from build123d import *

# Parameters (mm, degrees)
SKETCH2_W           = 200
SKETCH2_H           = 200
SKETCH2_R           = 60
BOSS_EXTRUDE1_DEPTH = 12
BOSS_EXTRUDE2_START = -2
SKETCH3_R           = 40
SKETCH3_R_2         = 26
BOSS_EXTRUDE2_DEPTH = 2


with BuildPart() as part:
    # Sketch1 → Revolve1 (revolve)
    with BuildSketch(Plane(origin=(0, 0, 0), x_dir=(-1, 0, 0), z_dir=(0, 0, -1)), mode=Mode.PRIVATE) as revolve1_sk:
        with BuildLine():
            Line((-40, 4), (-40, -8))
            Line((-40, -8), (-49.4043, -8))
            ThreePointArc((-49.4043, -8), (-52.5, -6.965718833), (-55.5957, -8))
            Line((-55.5957, -8), (-60, -8))
            Line((-60, -8), (-60, 4))
            Line((-60, 4), (-55.5957, 4))
            ThreePointArc((-55.5957, 4), (-52.5, 2.965718833), (-49.4043, 4))
            Line((-49.4043, 4), (-40, 4))
        make_face()
    revolve(revolve1_sk.sketch.rotate(Axis((0, 0, 0), (0, 1, 0)), 270), axis=Axis((0, 0, 0), (0, 1, 0)))

    # Sketch2 → Boss-Extrude1 (add)
    with BuildSketch(Plane(origin=(0, 4, 0), x_dir=(1, 0, 0), z_dir=(0, 1, 0))):
        Rectangle(SKETCH2_W, SKETCH2_H)
        Circle(SKETCH2_R, mode=Mode.SUBTRACT)
    extrude(amount=-BOSS_EXTRUDE1_DEPTH)

    # Sketch3 → Boss-Extrude2 (add)
    with BuildSketch(Plane(origin=(0, 4, 0), x_dir=(1, 0, 0), z_dir=(0, 1, 0)).offset(BOSS_EXTRUDE2_START)):
        with Locations(Location((0, 0, 0), (0, 0, 270))):
            Circle(SKETCH3_R)
        with Locations(Location((0, 0, 0), (0, 0, 270))):
            Circle(SKETCH3_R_2, mode=Mode.SUBTRACT)
    extrude(amount=BOSS_EXTRUDE2_DEPTH)


solid = part.part
CAD build for the part. Positions are in the model's coordinates, mm. A direction names the side the tool comes from. Give positions to 0.01 mm unless a question says otherwise; leave off trailing zeros. Loops run counter-clockwise (first coordinate to the right, second up) from the corner with the lowest first, then second, coordinate; pieces in that order, holes last. Notation, with made-up numbers: M 53,-25.75 L 101,-25.75 A23 ccw 101,-13.75 Z; hole C 82,5.5 d9. An arc over 180 degrees is marked long. One line per question, with ' | ' between items. Start each with the question number.
1. Saw through at B-B on z = 0. Give the cut face in (x, y).
2. Saw through at A-A on x = 0. Give the cut face in (y, z).
3. Saw through at C-C on y = -0.5. Give the cut face in (x, z), plus the area to 3 significant figures.
4. 3-axis set-ups, long thin cutter, end or side, ignore diameter. For faces 1 (the face through (-1, -2, 100)), 2 (the face through (-8, 2, 26)): which of +Z, -Z, +X, -X, +Y, -Y reach the whole face in a straight line?
5. Probe L1, parallel to X at y = 3.6, z = 0; L2, parallel to X at y = -7.5, z = -25; L3, parallel to X at y = -2.5, z = 0. List the from-to ranges inside material, lowest first. Write a range as from..to.
Result sheet:
1) outline: M -100,-8 L -55.6,-8 A5.15 cw -49.4,-8 L -40,-8 L -40,2 L -26,2 L -26,4 L -49.4,4 A5.15 cw -55.6,4 L -100,4 Z; M 26,2 L 40,2 L 40,-8 L 49.4,-8 A5.15 cw 55.6,-8 L 100,-8 L 100,4 L 55.6,4 A5.15 cw 49.4,4 L 26,4 Z
2) outline: M -8,-100 L 4,-100 L 4,-55.6 A5.15 cw 4,-49.4 L 4,-26 L 2,-26 L 2,-40 L -8,-40 L -8,-49.4 A5.15 cw -8,-55.6 Z; M -8,40 L 2,40 L 2,26 L 4,26 L 4,49.4 A5.15 cw 4,55.6 L 4,100 L -8,100 L -8,55.6 A5.15 cw -8,49.4 Z
3) outline: M -100,-100 L 100,-100 L 100,100 L -100,100 Z; hole C 0,0 d80 | area: 35,000 mm^2
4) face 1: +Z, +X, -X, +Y, -Y | face 2: -Y
5) L1: x = -100..-54.98, -50.02..-26, 26..50.02, 54.98..100 | L2: x = -100..-48.75, -43.55..-31.22, 31.22..43.55, 48.75..100 | L3: x = -100..-40, 40..100
